The listing builds one solid part. Answer for the finished solid, in the listing's coordinates (mm). Round coordinates to 2 decimals unless told otherwise and drop trailing zeros. Loops run counter-clockwise (first coordinate to the right, second up) from the corner with the lowest first, then second, coordinate; pieces in that order, holes last. Notation, with made-up numbers: M -36,-25.5 L -23,-25.5 A16 cw -23,-4.5 Z; hole C 18.25,-0.75 d10. An arc over 180 degrees is marked long. Put each result on its own line as item: value. Start each with the question number.
(1) Section B-B, the plane y = 0 is taken. Determine the outline of the cut face in (x, z) (3 decimals), then the cut area to 3 significant figures.
(2) Section C-C, the plane z = -7 is taken. Determine the outline of the cut face in (x, y) (3 decimals).
(3) Straight lines are drawn through the part: line 1 (Y direction, x = -2.2, z = 6.5); line 2 (Z direction, x = -2, y = 4.75); line 3 (Z direction, x = -2.8, y = 4.5). For each, find the intervals that lie inside material, in ascending order.
(4) Flat-ended cylindrical pins translate along their axes: P1, Ø3, axis at y = 3.175, z = 15.875, coming from the +X side; P2, Ø1, axis at x = -2, z = -10.5, coming from the -Y side. Find the tip coordinate at first contact, or state that the pin passes through.
(5) Determine the mould class of faces 1 (the face through (-1.565, 2.947, -14.137)), 2 (the face through (-1.565, 1.696, 18.685)), 3 (the face through (-2, 5, -19.05)), 4 (the face through (-2, -6.35, 0)) for opening direction Z: released by +Z, released by -Z, zero draft, split by the parting line, or undercut.
(6) Section D-D, the plane y = 2.5 is taken. Determine the outline of the cut face in (x, z) (3 decimals).
(7) Section A-A, the plane z = 0 is taken. Determine the outline of the cut face in (x, y) (3 decimals), then the cut area to 3 significant figures.
Autodesk Inventor part; units mm, degrees
ref_plane "YZ Plane" through (0, 0, 0) normal (1, 0, 0) x (0, 1, 0)
ref_plane "XZ Plane" through (0, 0, 0) normal (0, 1, 0) x (-1, 0, 0)
ref_plane "XY Plane" through (0, 0, 0) normal (0, 0, 1) x (1, 0, 0)
sketch "Sketch1" plane through (0, 0, 0) normal (1, 0, 0) x (0, 1, 0)
  line L0 (3.175, 6.35) -> (-3.175, 6.35) construction
  line L1 (-3.175, 6.35) -> (-3.175, -6.35) construction
  line L2 (-3.175, -6.35) -> (3.175, -6.35) construction
  line L3 (3.175, -6.35) -> (3.175, 6.35) construction
  line L4 (3.175, 6.35) -> (-3.175, -6.35) construction
  line L5 (-3.175, 6.35) -> (3.175, -6.35) construction
  circle A0 centre (0, 0) radius 1.5
  circle A1 centre (3.175, 6.35) radius 1.7526
  circle A2 centre (3.175, -6.35) radius 1.7526
  circle A3 centre (-3.175, 6.35) radius 1.7526
  circle A4 centre (-3.175, -6.35) radius 1.7526
  line L6 (6.35, 19.05) -> (-6.35, 19.05)
  line L7 (-6.35, 19.05) -> (-6.35, -19.05)
  line L8 (-6.35, -19.05) -> (6.35, -19.05)
  line L9 (6.35, -19.05) -> (6.35, 19.05)
  line L10 (6.35, 19.05) -> (-6.35, -19.05) construction
  line L11 (-6.35, 19.05) -> (6.35, -19.05) construction
  line L12 (-6.35, 0) -> (6.35, 0) construction
  line L13 (-6.35, -3.175) -> (6.35, -3.175)
  line L14 (6.35, 3.175) -> (-6.35, 3.175)
  arc A5 (-6.35, 3.175) -> (-6.35, -3.175) centre (-6.35, 0) ccw
  arc A6 (6.35, -3.175) -> (6.35, 3.175) centre (6.35, 0) ccw
  circle A7 centre (3.175, 15.875) radius 1.7526
  arc A8 (3.175, 19.05) -> (0.5332, 17.6362) centre (3.175, 15.875) ccw
  arc A9 (-5.8168, 8.1112) -> (-6.35, 6.35) centre (-3.175, 6.35) ccw
  line L15 (0.5332, 17.6362) -> (-5.8168, 8.1112)
  circle A10 centre (3.175, -15.875) radius 1.7526
  arc A11 (0.5332, -17.6362) -> (3.175, -19.05) centre (3.175, -15.875) ccw
  arc A12 (-6.35, -6.35) -> (-5.8168, -8.1112) centre (-3.175, -6.35) ccw
  line L16 (0.5332, -17.6362) -> (-5.8168, -8.1112)
  point P0 (3.175, -19.05)
  point P1 (-6.35, -6.35)
  dimension "d0" = 6.35
  dimension "d1" = 12.7
  dimension "d2" = 3
  dimension "d3" = 3.5052
  dimension "d6" = 12.7
  dimension "d9" = 6.35
  dimension "d12" = 12.7
  dimension "d13" = 38.1
  dimension "d14" = 6.35
  dimension "d20" = 3.5052
  dimension "d21" = 9.525
extrude "Extrusion2" add sketch "Sketch1" against normal blind 3.175 contours L9 L14 L7 A9 L15 A8 L6 | L9 L13 L7 L14 | L9 L8 A11 L16 A12 L7 L13
equation "\"d3\" = d20"
equation "\"d6\" = d1"
equation "\"d9\" = d0"
properties part number "Pin Cap" material "Aluminum 6061"
Recorded:
1. outline: M -3.175,-16.836 L 0,-16.836 L 0,-1.5 L -3.175,-1.5 Z; M -3.175,1.5 L 0,1.5 L 0,16.836 L -3.175,16.836 Z
1. area: 97.4 mm²
2. outline: M -3.175,-6.283 L 0,-6.283 L 0,-4.803 L -3.175,-4.803 Z; M -3.175,-1.547 L 0,-1.547 L 0,1.547 L -3.175,1.547 Z; M -3.175,4.803 L 0,4.803 L 0,6.35 L -3.175,6.35 Z
3. line 1: y = -6.35 to -4.92, -1.43 to 1.43, 4.92 to 6.35
3. line 2: z = -19.05 to -16.64, -15.11 to -7.12, -5.58 to 5.58, 7.12 to 15.11, 16.64 to 19.05
3. line 3: z = -19.05 to -17.02, -14.73 to -7.5, -5.2 to 5.2, 7.5 to 14.73, 17.02 to 19.05
4. P1: passes through
4. P2: stops at y = -4.56
5. face 1: undercut
5. face 2: released by +Z
5. face 3: released by -Z
5. face 4: zero draft
6. outline: M -3.175,-18.977 L 0,-18.977 L 0,-17.492 L -3.175,-17.492 Z; M -3.175,-14.258 L 0,-14.258 L 0,-7.967 L -3.175,-7.967 Z; M -3.175,-4.733 L 0,-4.733 L 0,4.733 L -3.175,4.733 Z; M -3.175,7.967 L 0,7.967 L 0,14.258 L -3.175,14.258 Z; M -3.175,17.492 L 0,17.492 L 0,18.977 L -3.175,18.977 Z
7. outline: M -3.175,-6.35 L 0,-6.35 L 0,-1.5 L -3.175,-1.5 Z; M -3.175,1.5 L 0,1.5 L 0,6.35 L -3.175,6.35 Z
7. area: 30.8 mm²
